Verification items for the finished model (mm, model axes). Round coordinates to 2 decimals unless told otherwise and drop trailing zeros. Write each loop counter-clockwise with the first axis right and the second up, starting at its lowest first coordinate (ties: lowest second). Pieces come first, ordered by that corner, then holes. Notation, with made-up numbers: (80, 9.5) -> (124, 9.5) arc R22 ccw to (124, 32.5) -> close; hole circle Ø5 at (30, 60). An arc over 180 degrees is marked (long way). Use CSV: the item, a comma, the result in double quotes.
Autodesk Fusion 360 part; units mm, degrees
sketch "Sketch1" plane through (0, 0, 0) normal (0, 1, 0) x (1, 0, 0)
  line L0 (-6.35, 25.4) -> (6.35, 25.4)
  line L1 (6.35, 25.4) -> (6.35, 0)
  line L2 (6.35, 0) -> (-6.35, 0)
  line L3 (-6.35, 0) -> (-6.35, 25.4)
  line L4 (-4, 25.4) -> (-4, 125)
  line L5 (-4, 125) -> (-2, 125)
  line L6 (-2, 125) -> (-2, 25.4)
  dimension "d1" = 25.4
  dimension "d2" = 12.7
  dimension "d5" = 125
  dimension "d6" = 2
  dimension "d12" = 2
extrude "Extrude1" add sketch "Sketch1" along normal mid plane 6.35 contours L0 L1 L2 L3
revolve "Revolve1" add sketch "Sketch1" angle 360 about axis through (-4, 0, -25.4) along (0, 0, -1) contours L0 L4 L5 L6
pattern_linear "R-Pattern1" count 3 spacing 4 along (1, 0, 0) of "Revolve1"
Q1. Mould release check, pull along X, two halves, no side actions. Record for faces 1 (the cylindrical face through (-5.6, -1.2, -74.5)), 2 (the flat face through (0, 0, -125)), 3 (the flat face through (-6.35, 0, -13)): released by +X, released by -X, zero draft, split by the parting line, or undercut.
Filled in:
face 1,"undercut"
face 2,"zero draft"
face 3,"released by -X"
Q2. Go/stop test with flat-tipped pins: P1, Ø5, axis at x = 3.5, z = -108, coming from the +Y side; P2, Ø2, axis at x = 3.5, z = -33, coming from the -Y side. Record where each tip stops, or that it passes through.
Filled in:
P1,"y = 2"
P2,"y = -2"
Q3. Section check A-A (x = 0). Record the cut outline in (y, z) (3 decimals).
Filled in:
outline,"(-3.175, -25.4) -> (-2, -25.4) -> (-2, -125) -> (2, -125) -> (2, -25.4) -> (3.175, -25.4) -> (3.175, 0) -> (-3.175, 0) -> close"
Q4. Material ranges on L1, parallel to X at y = -1, z = -116; L2, parallel to Z at x = -1.5, y = -1.5; L3, parallel to Y at x = 3.75, z = -82.5, recorded low to high.
Filled in:
L1,"-5.73 to -2.27, -1.73 to 1.73, 2.27 to 5.73"
L2,"-25.4 to 0"
L3,"-1.98 to 1.98"
